```python
from build123d import *

# Parameters (mm, degrees)
SKETCH1_W           = 5
SKETCH1_H           = 15
SKETCH1_H_2         = 5
SKETCH1_W_2         = 20
BOSS_EXTRUDE1_DEPTH = 10
SKETCH2_R           = 2.2
CUT_EXTRUDE1_DEPTH  = 10
SKETCH3_R           = 2.2
CUT_EXTRUDE2_DEPTH  = 10


with BuildPart() as part:
    # Sketch1 → Boss-Extrude1 (new body)
    with BuildSketch(Plane(origin=(0, 0, 0), x_dir=(0, 0, -1), z_dir=(1, 0, 0))):
        with Locations((2.5, 12.5)):
            Rectangle(SKETCH1_W, SKETCH1_H)
        with Locations((2.5, 2.5)):
            Rectangle(SKETCH1_W, SKETCH1_H_2)
        with Locations((15, 2.5)):
            Rectangle(SKETCH1_W_2, SKETCH1_H_2)
    extrude(amount=BOSS_EXTRUDE1_DEPTH)

    # Sketch2 → Cut-Extrude1 (cut)
    with BuildSketch(Plane(origin=(0, 0, -5), x_dir=(-1, 0, 0), z_dir=(0, 0, -1))):
        with Locations((-5, 13)):
            Circle(SKETCH2_R)
    extrude(amount=-CUT_EXTRUDE1_DEPTH, mode=Mode.SUBTRACT)

    # Sketch3 → Cut-Extrude2 (cut)
    with BuildSketch(Plane(origin=(0, 5, 0), x_dir=(1, 0, 0), z_dir=(0, 1, 0))):
        with Locations(Location((5, 20, 0), (0, 0, 270))):
            Circle(SKETCH3_R)
        with Locations(Location((5, 10, 0), (0, 0, 270))):
            Circle(SKETCH3_R)
    extrude(amount=-CUT_EXTRUDE2_DEPTH, mode=Mode.SUBTRACT)


solid = part.part
```
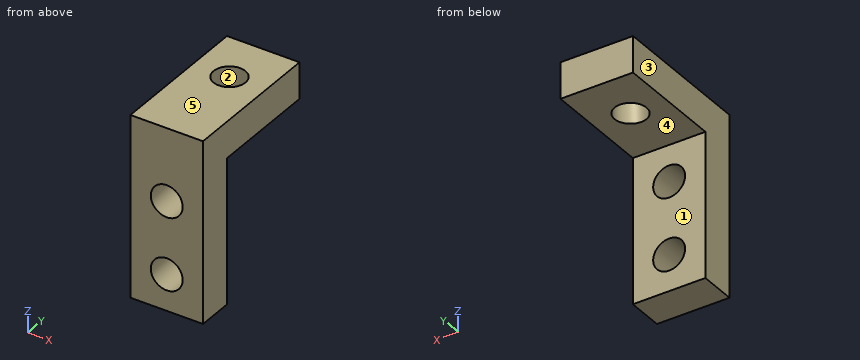
Could you check a few things on this model? Use its own coordinates, in mm. Face numbers are marked on the shaded views. A direction names the side the tool comes from. Coordinates: 2 decimals unless noted, no trailing zeros. Write each loop counter-clockwise with the first axis right and the second up, starting at its lowest first coordinate (ties: lowest second). Pieces come first, ordered by that corner, then holes. Notation, with made-up numbers: (25, 83) -> (71, 83) arc R25 ccw to (71, 97) -> close; hole circle Ø2 at (57, 4). An arc over 180 degrees is marked (long way). One line per question, with ' | ' between items. Start each with the question number.
1. If we section it at D-D (z = -4): Please give me the cut outline in (x, y).
2. If we section it at B-B (z = -10): Please give me the cut outline in (x, y), and give its area (3 significant figures).
3. For the marked faces 4 and 5, which set-ups out of +Z, -Z, +X, -X, +Y, -Y let a thin tool reach every point of the face, with its end or its side?
4. If we section it at A-A (y = 13): Please give me the cut outline in (x, z).
5. If we section it at C-C (x = 5): Please give me the cut outline in (y, z).
6. Will these pins go through, and if not, where does the flat tip stop? P1, Ø3.5, axis at x = 5, y = 13, coming from the +Z side; P2, Ø1.5, axis at x = 7.5, y = 10, coming from the -Z side; P3, Ø5, axis at x = 5, z = -10, coming from the +Y side.
7. Please list where these lines run through material, in increasing order: line 1 along X through (y, z) = (3, -20); line 2 along Z through (x, y) = (3, 3); line 3 along Y through (x, z) = (5, -1.9).
8. Thinking about a two-plate mould opening in X: for the marked faces 1, 2 and 3, which applies, pulls with the +X half, pulls with the -X half, needs draft (parallel to the pull), parting line crosses it, or undercut?
Return value:
1) outline: (0, 0) -> (10, 0) -> (10, 20) -> (0, 20) -> close; hole circle Ø4.4 at (5, 13)
2) outline: (0, 0) -> (2.8, 0) -> (2.8, 5) -> (0, 5) -> close; (7.2, 0) -> (10, 0) -> (10, 5) -> (7.2, 5) -> close | area: 28.0 mm²
3) face 4: -Z, +X, -X, +Y | face 5: +Z, +X, -X, +Y, -Y
4) outline: (0, -5) -> (2.8, -5) -> (2.8, 0) -> (0, 0) -> close; (7.2, -5) -> (10, -5) -> (10, 0) -> (7.2, 0) -> close
5) outline: (0, -25) -> (5, -25) -> (5, -22.2) -> (0, -22.2) -> close; (0, -17.8) -> (5, -17.8) -> (5, -12.2) -> (0, -12.2) -> close; (0, -7.8) -> (5, -7.8) -> (5, -5) -> (10.8, -5) -> (10.8, 0) -> (0, 0) -> close; (15.2, -5) -> (20, -5) -> (20, 0) -> (15.2, 0) -> close
6) P1: passes through | P2: stops at z = -5 | P3: stops at y = 5
7) line 1: x = 0 to 2.8, 7.2 to 10 | line 2: z = -25 to -20.92, -19.08 to -10.92, -9.08 to 0 | line 3: y = 0 to 10.8, 15.2 to 20
8) face 1: needs draft | face 2: undercut | face 3: pulls with the -X half
